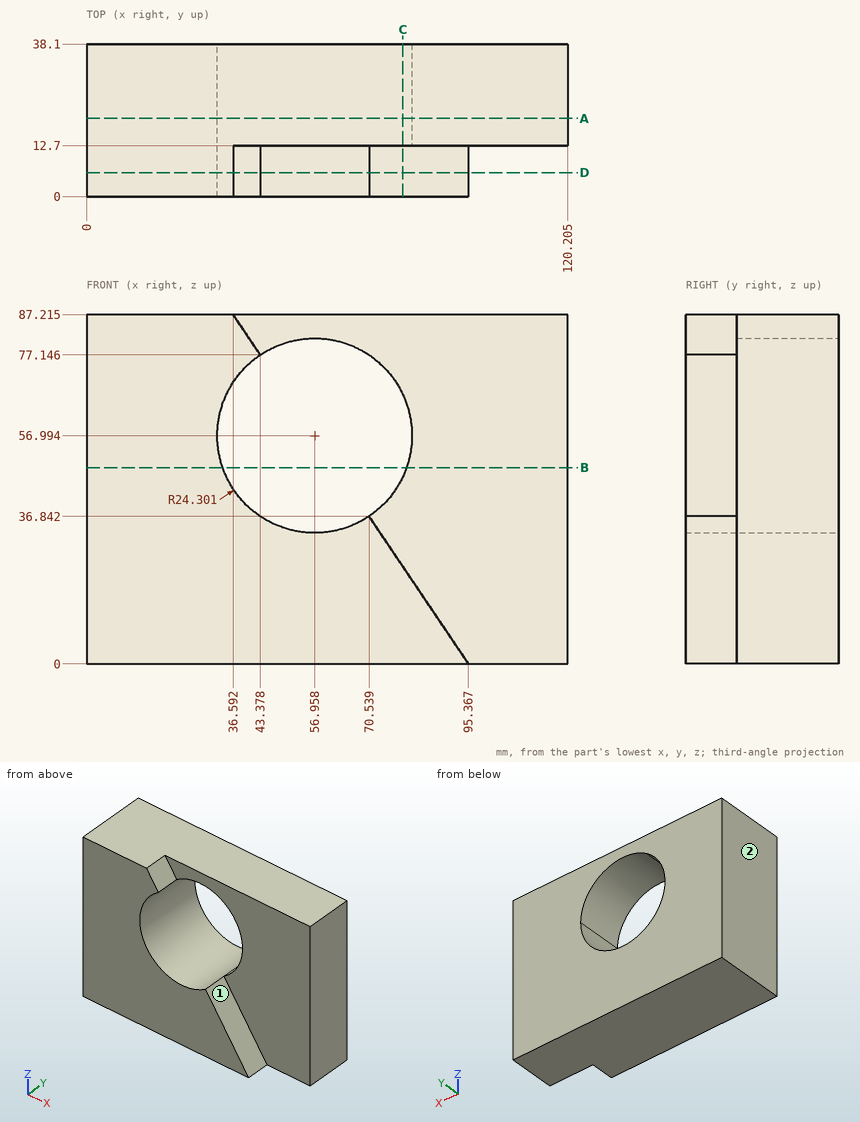
Print and shaded views of the part. All mm, measured from the part's lowest x, y and z. A direction names the side the tool comes from. Coordinates: 2 decimals unless noted, no trailing zeros. Loops run counter-clockwise (first coordinate to the right, second up) from the corner with the lowest first, then second, coordinate; pieces in that order, holes last. Notation, with made-up numbers: (-35, -16) - (-17, -16) arc R13 ccw to (-17, 9) - close; hole circle Ø4 at (33, 86.25). An arc over 180 degrees is marked (long way). Write item = value, one per line. Start each with the question number.
Item 1: Wall check: L1, parallel to Y at x = 114.5, z = 8; L2, parallel to X at y = 35.5, z = 36 (1 decimal); L3, parallel to X at y = 17.5, z = 50 (1 decimal). Give the ranges that are in metal, low to high. Write a range as from..to.
Item 2: Cut at C-C, the plane x = 79. Give the cut face in (y, z) (1 decimal).
Item 3: Flat gauge pins, fed straight in: pin 1 Ø5 at (x, z) = (90.5, 28) entering from -Y; pin 2 Ø5 at (y, z) = (17.5, 69) entering from -X; pin 3 Ø1.5 at (x, y) = (63.5, 9.5) entering from +Z; pin 4 Ø6 at (y, z) = (4, 64.5) entering from +X (1 decimal). Where does each tip first touch, or does it go through?
Item 4: 3-axis set-ups, long thin cutter, end or side, ignore diameter. For the marked faces 1 and 2: which of +Z, -Z, +X, -X, +Y, -Y reach the whole face in a straight line?
Item 5: Cut at A-A, the plane y = 19.5. Give the cut face in (x, z) (1 decimal).
Item 6: Cut at B-B, the plane z = 49. Give the cut face in (x, y) (1 decimal), and give its area (3 significant figures).
Item 7: Cut at D-D, the plane y = 6. Give the cut face in (x, z) (1 decimal).
The answers:
q1.L1 = 12.7..38.1
q1.L2 = 0..44.7, 69.2..120.2
q1.L3 = 0..33.7, 80.2..120.2
q2.outline = (0, 0) - (38.1, 0) - (38.1, 46.8) - (12.7, 46.8) - (12.7, 24.3) - (0, 24.3) - close; (12.7, 67.2) - (38.1, 67.2) - (38.1, 87.2) - (12.7, 87.2) - close
q3.pin_1 = 12.7
q3.pin_2 = 0
q3.pin_3 = 33.81
q3.pin_4 = 35
q4.face_1 = +Z, +X, -Y
q4.face_2 = +Z, -Z, -X, +Y, -Y
q5.outline = (0, 0) - (120.2, 0) - (120.2, 87.2) - (0, 87.2) - close; hole (70.5, 36.8) arc R24.3 ccw to (81.3, 57) arc R24.3 ccw (long way) to start
q6.outline = (0, 0) - (34, 0) - (34, 38.1) - (0, 38.1) - close; (79.9, 12.7) - (120.2, 12.7) - (120.2, 38.1) - (79.9, 38.1) - close
q6.area = 2,320 mm2
q7.outline = (0, 0) - (95.4, 0) - (70.5, 36.8) arc R24.3 cw to (43.4, 77.1) - (36.6, 87.2) - (0, 87.2) - close
